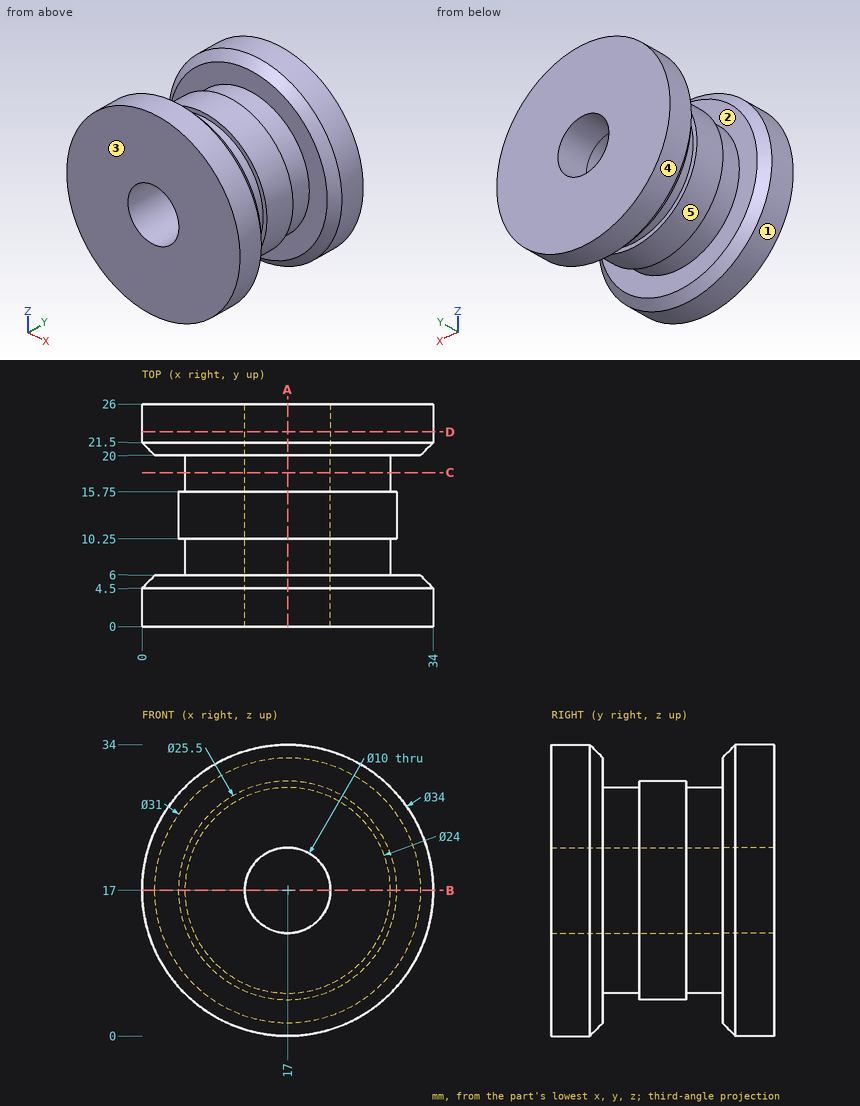
Can you work these out from the drawing? Everything is in mm from the part's minimum corner. A direction names the side the tool comes from. Give positions to 0.01 mm unless a question says otherwise; leave off trailing zeros. Order: outer loops, then holes, each group sorted by start corner. A loop starts at its lowest first (then second) coordinate and runs counter-clockwise, first axis right, second up. Notation, with made-up numbers: M 12,-19 L 36,-19 A7 cw 36,-11 Z; hole C 58,69 d6. An arc over 180 degrees is marked long. One line per question, with ' | ' between items.
1. I want a section at B-B (z = 17). List the corners of the cut face in (x, y) for me.
Results:
outline: M 0,0 L 12,0 L 12,26 L 0,26 L 0,21.5 L 1.5,20 L 5,20 L 5,15.75 L 4.25,15.75 L 4.25,10.25 L 5,10.25 L 5,6 L 1.5,6 L 0,4.5 Z; M 22,0 L 34,0 L 34,4.5 L 32.5,6 L 29,6 L 29,10.25 L 29.75,10.25 L 29.75,15.75 L 29,15.75 L 29,20 L 32.5,20 L 34,21.5 L 34,26 L 22,26 Z
2. We'd pull the mould along Y, two halves only. Please class the marked faces 1, 2 and 3: +Y half, -Y half, draft (parallel to the pull), parting line (faces both ways), or undercut.
Results:
face 1: draft | face 2: undercut | face 3: -Y half
3. I want a section at A-A (x = 17). List the corners of the cut face in (y, z) for me, and give its area (3 significant figures).
Results:
outline: M 0,0 L 4.5,0 L 6,1.5 L 6,5 L 10.25,5 L 10.25,4.25 L 15.75,4.25 L 15.75,5 L 20,5 L 20,1.5 L 21.5,0 L 26,0 L 26,12 L 0,12 Z; M 0,22 L 26,22 L 26,34 L 21.5,34 L 20,32.5 L 20,29 L 15.75,29 L 15.75,29.75 L 10.25,29.75 L 10.25,29 L 6,29 L 6,32.5 L 4.5,34 L 0,34 Z | area: 488 mm²
4. If I drill on line 1 (Z direction, x = 17, y = 9.25); line 2 (Y direction, x = 16, z = 31); line 3 (Z direction, x = 19, y = 21), over which ranges is the centre line in solid material (lowest first)?
Results:
line 1: 5 to 12, 22 to 29 | line 2: 0 to 6, 20 to 26 | line 3: 0.62 to 12.42, 21.58 to 33.38
5. I'm going to push flat-ended pins straight in: pin 1 (6 mm diameter, centred on x = 17, z = 17, fed in from -Y); pin 2 (8 mm diameter, centred on y = 22.5, z = 24, fed in from +X); pin 3 (10 mm diameter, centred on y = 9, z = 11.5, fed in from -X); pin 4 (12 mm diameter, centred on x = 28.5, y = 4, fed in from -Z). Where does each tip first touch, or does it pass through?
Results:
pin 1: through | pin 2: x = 33.73 | pin 3: x = 0.33 | pin 4: z = 0.91
6. I want a section at C-C (y = 18). List the corners of the cut face in (x, z) for me.
Results:
outline: C 17,17 d24; hole C 17,17 d10
7. For the marked faces 4 and 5, which set-ups out of +Z, -Z, +X, -X, +Y, -Y let a thin tool reach every point of the face, with its end or its side?
Results:
face 4: +Y, -Y | face 5: none
8. I want a section at D-D (y = 22.75). List the corners of the cut face in (x, z) for me.
Results:
outline: C 17,17 d34; hole C 17,17 d10
